```python
from build123d import *

# Parameters (mm, degrees)
BOSS_EXTRUDE1_DEPTH = 10
SKETCH2_R           = 1.5
CUT_EXTRUDE1_DEPTH  = 8
SKETCH3_R           = 3
CUT_EXTRUDE2_DEPTH  = 24.505318713


with BuildPart() as part:
    # Sketch1 → Boss-Extrude1 (new body)
    with BuildSketch(Plane(origin=(0, 0, 0), x_dir=(1, 0, 0), z_dir=(0, 1, 0))):
        with BuildLine():
            ThreePointArc((-12.5, 0), (0, 12.5), (12.5, 0))
            Line((12.5, 0), (18.5, 0))
            ThreePointArc((18.5, 0), (0, 18.5), (-18.5, 0))
            Line((-18.5, 0), (-12.5, 0))
        make_face()
    extrude(amount=BOSS_EXTRUDE1_DEPTH)

    # Sketch2 → Cut-Extrude1 (cut)
    with BuildSketch(Plane.XY):
        with Locations((-15.5, 5)):
            Circle(SKETCH2_R)
    cut_extrude1 = extrude(amount=-CUT_EXTRUDE1_DEPTH, mode=Mode.SUBTRACT)

    # Sketch3 → Cut-Extrude2 (cut, through all)
    with BuildSketch(Plane.XY.offset(-8)):
        with Locations((-15.5, 5)):
            Circle(SKETCH3_R)
    cut_extrude2 = extrude(amount=-CUT_EXTRUDE2_DEPTH, mode=Mode.SUBTRACT)

    # Mirror1: Cut-Extrude1, Cut-Extrude2 across plane
    add(cut_extrude1.mirror(Plane(origin=(0, 0, 0), x_dir=(0, 0, 1), z_dir=(1, 0, 0))), mode=Mode.SUBTRACT)
    add(cut_extrude2.mirror(Plane(origin=(0, 0, 0), x_dir=(0, 0, 1), z_dir=(1, 0, 0))), mode=Mode.SUBTRACT)


solid = part.part
```
Check sheet for the modelled part. Datum: model origin and axes. Units: mm. A direction names the side the tool comes from. Round coordinates to 2 decimals unless told otherwise and drop trailing zeros. Write each loop counter-clockwise with the first axis right and the second up, starting at its lowest first coordinate (ties: lowest second). Pieces come first, ordered by that corner, then holes. Notation, with made-up numbers: M 46.25,78 L 60.25,78 A21 cw 60.25,105 Z; hole C -14,51 d5. An arc over 180 degrees is marked long. Write item = value, one per line. Start each with the question number.
1. Section check C-C, the plane x = -16. Record the cut outline in (y, z).
2. Release check for a two-part mould opening along X. For faces 1 (the cylindrical face through (0.407, 4.93, -18.496)), 2 (the flat face through (-17, 4, 0)), 3 (the cylindrical face through (14.114, 4.425, -3.944)) record: pulls with the +X half, pulls with the -X half, needs draft (parallel to the pull), parting line crosses it, or undercut.
3. Section check A-A, the plane z = -2.5. Record the cut outline in (x, y), then the cut area to 3 significant figures.
4. Gauge pin test, flat ends, axial feed: pin 1 (3.5 mm diameter, centred on x = -15, y = 4.5, fed in from -Z); pin 2 (2 mm diameter, centred on x = -6.5, y = 6.5, fed in from -Z); pin 3 (1.5 mm diameter, centred on y = 8, z = -10, fed in from -X). Record the tip position at first contact, or that the pin passes through.
5. Tool access check on faces 4 (the flat face through (0, 0, -13)), 5 (the cylindrical face through (-12.5, 4.9, -10.2)). Record the directions out of +Z, -Z, +X, -X, +Y, -Y that give a thin tool (end or side, any length) a straight path to the whole face; none if there is none.
6. Section check D-D, the plane z = -13. Record the cut outline in (x, y).
7. Section check B-B, the plane y = 5. Record the cut outline in (x, z).
8. Scan lines: line 1 (Y direction, x = -15.5, z = -3.25); line 2 (Y direction, x = -15.5, z = -9.7); line 3 (X direction, y = 5, z = -3). Record each from-to range of solid material in increasing order. Write a range as [from, to].
Results found:
q1.outline = M 0,-9.29 L 2.04,-9.29 L 2.04,-8 L 3.59,-8 L 3.59,0 L 0,0 Z; M 6.41,-8 L 7.96,-8 L 7.96,-9.29 L 10,-9.29 L 10,0 L 6.41,0 Z
q2.face_1 = parting line crosses it
q2.face_2 = needs draft
q2.face_3 = undercut
q3.outline = M -18.33,0 L -12.25,0 L -12.25,10 L -18.33,10 Z; M 12.25,0 L 18.33,0 L 18.33,10 L 12.25,10 Z; hole C -15.5,5 d3; hole C 15.5,5 d3
q3.area = 108 mm^2
q4.pin_1 = -8
q4.pin_2 = -17.66
q4.pin_3 = -16.02
q5.face_4 = +Z, -Z, +X, -X, -Y
q5.face_5 = -Z
q6.outline = M -13.16,0 L 13.16,0 L 13.16,3.12 A3 cw 13.16,6.88 L 13.16,10 L -13.16,10 L -13.16,6.88 A3 cw -13.16,3.12 Z
q7.outline = M -18.5,0 A18.5 ccw -17,-7.3 L -17,0 Z; M -14,-8 L -12.5,-8 L -12.5,-13.64 A18.5 ccw 12.5,-13.64 L 12.5,-8 L 14,-8 L 14,0 L 12.5,0 A12.5 cw -12.5,0 L -14,0 Z; M 17,-7.3 A18.5 ccw 18.5,0 L 17,0 Z
q8.line_1 = [0, 3.5], [6.5, 10]
q8.line_2 = [0, 2], [8, 10]
q8.line_3 = [-18.26, -17], [-14, -12.13], [12.13, 14], [17, 18.26]
